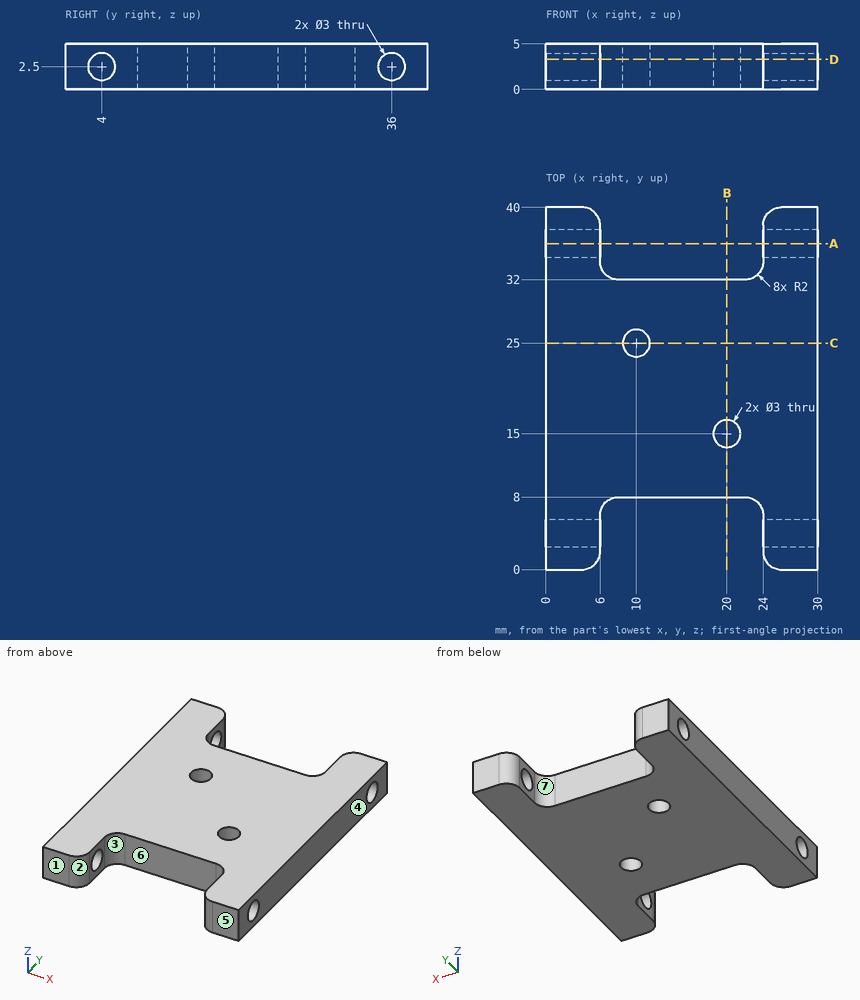
Drawing for the job (mm, zero at the part's lowest x, y, z). A direction names the side the tool comes from. Give positions to 0.01 mm unless a question says otherwise; leave off trailing zeros. Order: outer loops, then holes, each group sorted by start corner. A loop starts at its lowest first (then second) coordinate and runs counter-clockwise, first axis right, second up. Notation, with made-up numbers: (72.25, 27) - (123.25, 27) arc R27 ccw to (123.25, 52) - close; hole circle Ø4 at (70, 12.5). An arc over 180 degrees is marked (long way). Use one line per item in the form item = value.
Item 1: Which spindle directions (+Z, -Z, +X, -X, +Y, -Y) get a long thin tool onto all of the face, cutting with end or side? Do the marked faces 5, 6 and 7. Say none if no direction does.
Solution:
face_5 = +Z, -Z, +X, -X, -Y
face_6 = +Z, -Z, -Y
face_7 = +Z, -Z, +Y
Item 2: Pin check, flat tips, straight feed: pin 1 Ø2 at (x, z) = (9.5, 4) entering from -Y; pin 2 Ø1.5 at (x, z) = (12.5, 1.5) entering from +Y. Stop position of each tip, or through.
Solution:
pin_1 = 8
pin_2 = 32
Item 3: Two-plate mould, pull along X, no slides. Class the marked faces 1, 2, 3 and 4: released by +X, released by -X, zero draft, split by the parting line, or undercut.
Solution:
face_1 = zero draft
face_2 = undercut
face_3 = undercut
face_4 = released by +X
Item 4: Slice it at C-C on y = 25. Give the cut face in (x, z).
Solution:
outline = (0, 0) - (8.5, 0) - (8.5, 5) - (0, 5) - close; (11.5, 0) - (30, 0) - (30, 5) - (11.5, 5) - close
Item 5: Slice it at D-D on z = 3.3. Count the separate pieces of the cut face and the enclosed holes in it, and give its area (3 significant figures).
Solution:
separate_pieces = 5
enclosed_holes = 2
area = 837 mm2
Item 6: Slice it at A-A on y = 36. Give the cut face in (x, z).
Solution:
outline = (0, 0) - (6, 0) - (6, 1) - (0, 1) - close; (0, 4) - (6, 4) - (6, 5) - (0, 5) - close; (24, 0) - (30, 0) - (30, 1) - (24, 1) - close; (24, 4) - (30, 4) - (30, 5) - (24, 5) - close
Item 7: Probe probe 1 along X at (y, z) = (36, 4.55); probe 2 along Z at (x, y) = (25.9, 4); probe 3 along Y at (x, z) = (25.25, 1.8). List the from-to ranges inside material, lowest first. Write a range as from..to.
Solution:
probe_1 = 0..6, 24..30
probe_2 = 0..1, 4..5
probe_3 = 0.15..2.67, 5.33..34.67, 37.33..39.85
Item 8: Slice it at B-B on x = 20. Give the cut face in (y, z).
Solution:
outline = (8, 0) - (13.5, 0) - (13.5, 5) - (8, 5) - close; (16.5, 0) - (32, 0) - (32, 5) - (16.5, 5) - close
